from build123d import *

# Parameters (mm, degrees)
BOSS_EXTRUDE1_DEPTH = 0.625
SKETCH2_R           = 1
CUT_EXTRUDE1_DEPTH  = 2
SCALE1_SCALE        = 0.6


with BuildPart() as part:
    # Sketch1 → Boss-Extrude1 (new body)
    with BuildSketch(Plane(origin=(0, 0, 0), x_dir=(1, 0, 0), z_dir=(0, 1, 0))):
        with BuildLine():
            Line((8.997858244, 0.196333965), (9.848841271, -38.803666035))
            ThreePointArc((9.848841271, -38.803666035), (9.449049837, -40.366651199), (8.297497314, -41.496555))
            ThreePointArc((8.297497314, -41.496555), (5.081486735, -44.617860887), (3.9, -48.940980546))
            Line((3.9, -48.940980546), (3.9, -75.940980546))
            ThreePointArc((3.9, -75.940980546), (3.144994432, -77.930955421), (1.26, -78.919302221))
            ThreePointArc((1.26, -78.919302221), (-6.994111479, -76.326677148), (-10.499709039, -68.417009214))
            ThreePointArc((-10.499709039, -68.417009214), (-3.259075008, -58.361278544), (-0.7, -46.237102878))
            Line((-0.7, -46.237102878), (-0.7, -18.987102878))
            ThreePointArc((-0.7, -18.987102878), (-2.95691693, -11.364767277), (-9, -6.2))
            Line((-9, -6.2), (-9, 0))
            ThreePointArc((-9, 0), (-0.098172823, 8.999464545), (8.997858244, 0.196333965))
        make_face()
    extrude(amount=BOSS_EXTRUDE1_DEPTH)

    # Sketch2 → Cut-Extrude1 (cut)
    with BuildSketch(Plane(origin=(0, 0.625, 0), x_dir=(1, 0, 0), z_dir=(0, 1, 0))):
        with Locations(Location((-2.716354086, -71.695176359, 0), (0, 0, 270))):
            Circle(SKETCH2_R)
    extrude(amount=-CUT_EXTRUDE1_DEPTH, mode=Mode.SUBTRACT)


with BuildPart() as part_1:
    # Scale1: scaled about (1.258353423, 0.3125, 30.69527069)
    add(part.part.scale(SCALE1_SCALE).moved(Location((0.503341369, 0.125, 12.278108276))))


solid = part_1.part
Check sheet for the modelled part. Datum: model origin and axes. Units: mm. A direction names the side the tool comes from. Coordinates: 2 decimals unless noted, no trailing zeros. Write each loop counter-clockwise with the first axis right and the second up, starting at its lowest first coordinate (ties: lowest second). Pieces come first, ordered by that corner, then holes.
Item 1: Cross-section at B-B on y = 0.35. Record the boundary of the cut face in (x, z).
Numbers:
outline: (-5.8, 53.33) arc R18 cw to (0.08, 40.02) - (0.08, 23.67) arc R8.4 cw to (-4.9, 16) - (-4.9, 12.28) arc R5.4 ccw to (5.9, 12.16) - (6.41, 35.56) arc R1.8 ccw to (5.48, 37.18) arc R5.1 cw to (2.84, 41.64) - (2.84, 57.84) arc R1.8 ccw to (1.26, 59.63) arc R6.3 ccw to start; hole circle Ø1.2 at (-1.13, 55.3)
Item 2: Cross-section at A-A on x = -2.5. Record the boundary of the cut face in (y, z) (3 decimals).
Numbers:
outline: (0.125, 7.79) - (0.5, 7.79) - (0.5, 17.61) - (0.125, 17.61) - close; (0.125, 49.312) - (0.5, 49.312) - (0.5, 58.913) - (0.125, 58.913) - close
Item 3: Cross-section at D-D on x = 4.5. Record the boundary of the cut face in (y, z) (3 decimals), then the cut area to 3 significant figures.
Numbers:
outline: (0.125, 8.647) - (0.5, 8.647) - (0.5, 37.881) - (0.125, 37.881) - close
area: 11.0 mm2
Item 4: Scan lines: probe 1 along X at (y, z) = (0.2, 39.5); probe 2 along Z at (x, y) = (-3, 0.4); probe 3 along Z at (x, y) = (-4.25, 0.45). Record each from-to range of solid material in increasing order.
Numbers:
probe 1: x = 0.08 to 3.32
probe 2: z = 8.17 to 17.17, 50.09 to 58.61
probe 3: z = 9.72 to 16.32, 51.73 to 57.51
Item 5: Depth check by flat-ended pin: pin 1 Ø1.6 at (x, z) = (-1.13, 55.3) entering from -Y (3 decimals). Enter the tip coordinate at first touch or a pass-through.
Numbers:
pin 1: stops at y = 0.125
Item 6: Mould release check, pull along Z, two halves, no side actions. Record for faces 1 (the face through (2, 0.5, 27)), 2 (the face through (0.33, 0.31, 6.88)), 3 (the face through (-1.36, 0.32, 55.85)): released by +Z, released by -Z, zero draft, split by the parting line, or undercut.
Numbers:
face 1: zero draft
face 2: released by -Z
face 3: undercut
Item 7: Access from +Z, -Z, +X, -X, +Y, -Y to the whole of each face (thin tool, end or side, straight path). Record for faces 4 (the face through (2, 0.125, 27)), 5 (the face through (-1.5, 0.3, 47.4)).
Numbers:
face 4: +Z, -Z, +X, -X, -Y
face 5: -X, +Y, -Y
Item 8: Cross-section at C-C on z = 54. Record the boundary of the cut face in (x, y) (3 decimals), then the cut area to 3 significant figures.
Numbers:
outline: (-5.766, 0.125) - (2.843, 0.125) - (2.843, 0.5) - (-5.766, 0.5) - close
area: 3.23 mm2
